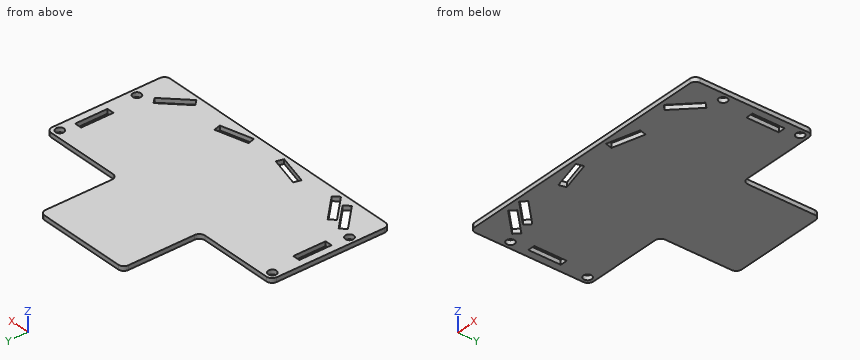
Autodesk Inventor part; units mm, degrees
ref_plane "YZ Plane" through (0, 0, 0) normal (1, 0, 0) x (0, 1, 0)
ref_plane "XZ Plane" through (0, 0, 0) normal (0, 1, 0) x (-1, 0, 0)
ref_plane "XY Plane" through (0, 0, 0) normal (0, 0, 1) x (1, 0, 0)
sketch "Szkic1" plane through (0, 0, 0) normal (0, 0, 1) x (1, 0, 0)
  circle A0 centre (-2, -7.4599) radius 1.4
  circle A1 centre (-2, 20.4244) radius 1.4
  circle A2 centre (-95, -7.4599) radius 1.4
  circle A3 centre (-95, 20.4244) radius 1.4
  line L0 (-98.5, 23.9244) -> (-98.5, -20.9244)
  line L1 (-97.6, 23.9244) -> (-97.6, -20.9244)
  line L2 (-98.5, -20.9244) -> (-91.5, -20.9244)
  line L3 (-98.5, 23.9244) -> (-91.5, 23.9244)
  line L4 (-98.5, -19.9244) -> (-91.5, -19.9244)
  line L5 (-91.5, -7.4599) -> (-91.5, -20.9244)
  line L6 (-97.6, 23.0244) -> (-92.3999, 23.0244)
  line L7 (-48.5, -51.6271) -> (-48.5, 68.0164)
  line L8 (-97.6, -19.9244) -> (-48.5, -19.9244)
  line L9 (-48.5, -19.9244) -> (-48.5, 23.0244)
  line L10 (-48.5, 23.0244) -> (-97.6, 23.0244)
  line L11 (-97.6, 23.0244) -> (-97.6, -19.9244)
  line L12 (0.6, -19.9244) -> (-48.5, -19.9244)
  line L13 (-48.5, 23.0244) -> (0.6, 23.0244)
  line L14 (0.6, 23.0244) -> (0.6, -19.9244)
  point P0 (0, 0)
  dimension "d0" = 0.9
  dimension "d1" = 1
  dimension "d2" = 0.9
extrude "Wyciągnięcie proste1" add sketch "Szkic1" along normal blind 1.6 contours L1 L6 L10 L7 L8 L4 | L7 L13 L14 L12
sketch "Szkic2" plane through (0, 0, 1.6) normal (0, 0, 1) x (1, 0, 0)
  line L0 (-29.5, 25.9244) -> (-29.5, 36.1286)
  line L1 (-31.5, 51.9244) -> (-65.5, 51.9244)
  line L2 (-67.5, 36.1286) -> (-67.5, 25.9244)
  line L3 (0.6, 23.0244) -> (-97.6, 23.0244)
  line L4 (-29.5, 23.0244) -> (-67.5, 23.0244)
  line L5 (-67.5, 23.0244) -> (-67.5, 51.9244)
  line L6 (-67.5, 51.9244) -> (-29.5, 51.9244)
  line L7 (-29.5, 51.9244) -> (-29.5, 23.0244)
  line L8 (-30.4, 23.9244) -> (-66.6, 23.9244)
  line L9 (-66.6, 23.9244) -> (-66.6, 51.0244)
  line L10 (-66.6, 51.0244) -> (-30.4, 51.0244)
  line L11 (-30.4, 51.0244) -> (-30.4, 23.9244)
  line L12 (-30.4, 23.9244) -> (-30.4, 23.0244)
  line L13 (-66.6, 23.9244) -> (-66.6, 23.0244)
  point P0 (0, 0)
  point P1 (-67.5, 37.4744)
  point P2 (-29.5, 37.4744)
  point P3 (-29.5, 31.0265)
  point P4 (-48.5, 51.9244)
  dimension "d5" = 0.9
extrude "Wyciągnięcie proste2" add sketch "Szkic2" against normal blind 1.6 contours L3 L13 L8 L12 | L8 L9 L10 L11
sketch "Szkic3" plane through (0, 0, 1.6) normal (0, 0, 1) x (1, 0, 0)
  line L0 (-94.4, -0.5756) -> (-94.4, 10.1244)
  line L1 (-94.4, 10.1244) -> (-92.8, 10.1244)
  line L2 (-92.8, 10.1244) -> (-92.8, -0.5756)
  line L3 (-94.4, -0.5756) -> (-92.8, -0.5756)
  line L4 (-77.7433, -17.9244) -> (-76.6119, -16.7931)
  line L5 (-77.7433, -17.9244) -> (-85.3094, -10.3584)
  line L6 (-84.178, -9.227) -> (-76.6119, -16.7931)
  line L7 (-85.3094, -10.3584) -> (-84.178, -9.227)
  line L8 (-63.3019, -13.6096) -> (-52.9665, -16.379)
  line L9 (-63.716, -15.1551) -> (-63.3019, -13.6096)
  line L10 (-53.3806, -17.9244) -> (-63.716, -15.1551)
  line L11 (-29.1305, -15.1551) -> (-39.4659, -17.9244)
  line L12 (-39.88, -16.379) -> (-29.5446, -13.6096)
  line L13 (-29.1305, -15.1551) -> (-29.5446, -13.6096)
  line L14 (-39.4659, -17.9244) -> (-39.88, -16.379)
  line L15 (-53.3806, -17.9244) -> (-52.9665, -16.379)
  line L16 (-14.4607, -17.9244) -> (-15.592, -16.7931)
  line L17 (-15.592, -16.7931) -> (-8.026, -9.227)
  line L18 (-6.8946, -10.3584) -> (-14.4607, -17.9244)
  line L19 (-6.8946, -10.3584) -> (-8.026, -9.227)
  line L20 (-2.6, 14.4244) -> (-4.2, 14.4244)
  line L21 (-4.2, 3.7244) -> (-4.2, 14.4244)
  line L22 (-2.6, 3.7244) -> (-4.2, 3.7244)
  line L23 (-2.6, 14.4244) -> (-2.6, 3.7244)
  line L24 (-92.3, -1.0756) -> (-92.3, 10.6244)
  line L25 (-92.3, 10.6244) -> (-94.9, 10.6244)
  line L26 (-94.9, 10.6244) -> (-94.9, -1.0756)
  line L27 (-94.9, -1.0756) -> (-92.3, -1.0756)
  line L28 (-75.9048, -16.7931) -> (-77.7433, -18.6316)
  line L29 (-77.7433, -18.6316) -> (-86.0165, -10.3584)
  line L30 (-86.0165, -10.3584) -> (-84.178, -8.5199)
  line L31 (-84.178, -8.5199) -> (-75.9048, -16.7931)
  line L32 (-52.3541, -16.0254) -> (-63.6554, -12.9972)
  line L33 (-63.6554, -12.9972) -> (-64.3284, -15.5086)
  line L34 (-64.3284, -15.5086) -> (-53.027, -18.5368)
  line L35 (-53.027, -18.5368) -> (-52.3541, -16.0254)
  line L36 (-29.1911, -12.9972) -> (-40.4924, -16.0254)
  line L37 (-40.4924, -16.0254) -> (-39.8195, -18.5368)
  line L38 (-39.8195, -18.5368) -> (-28.5181, -15.5086)
  line L39 (-28.5181, -15.5086) -> (-29.1911, -12.9972)
  line L40 (-8.026, -8.5199) -> (-16.2991, -16.7931)
  line L41 (-16.2991, -16.7931) -> (-14.4607, -18.6316)
  line L42 (-14.4607, -18.6316) -> (-6.1875, -10.3584)
  line L43 (-6.1875, -10.3584) -> (-8.026, -8.5199)
  line L44 (-4.7, 3.2244) -> (-4.7, 14.9244)
  line L45 (-4.7, 14.9244) -> (-2.1, 14.9244)
  line L46 (-2.1, 14.9244) -> (-2.1, 3.2244)
  line L47 (-2.1, 3.2244) -> (-4.7, 3.2244)
  point P0 (0, 0)
  dimension "d8" = 0.5
  dimension "d9" = 0.5
  dimension "d10" = 0.5
  dimension "d11" = 0.5
  dimension "d12" = 0.5
  dimension "d13" = 0.5
extrude "Wyciągnięcie proste3" cut sketch "Szkic3" against normal blind 1.6 contours L0 L1 L2 L3 | L5 L7 L6 L4 | L8 L15 L10 L9 | L11 L14 L12 L13 | L16 L17 L19 L18 | L23 L22 L21 L20 | L27 L26 L25 L24 | L28 L29 L30 L31 | L35 L34 L33 L32 | L39 L38 L37 L36 | L43 L42 L41 L40 | L44 L45 L46 L47
fillet "Zaokrąglenie1" radius 2 8 edges at (-66.6, 51.0244, 0.8) (-66.6, 23.0244, 0.8) (-97.6, 23.0244, 0.8) (-97.6, -19.9244, 0.8) (0.6, 23.0244, 0.8) (0.6, -19.9244, 0.8) (-30.4, 23.0244, 0.8) (-30.4, 51.0244, 0.8)
sketch "Szkic4" plane through (0, 0, 1.6) normal (0, 0, 1) x (1, 0, 0)
  circle A0 centre (-2, 20.4244) radius 1.4
  circle A1 centre (-2, -7.4599) radius 1.4
  circle A2 centre (-95, 20.4244) radius 1.4
  circle A3 centre (-95, -7.4599) radius 1.4
  point P0 (0, 0)
hole "Otwór1" at (-2, 20.4244, 1.6) at (-2, -7.4599, 1.6) at (-95, 20.4244, 1.6) at (-95, -7.4599, 1.6) direction (0, 0, -1) diameter 3 end through all
sketch "Szkic5" plane through (0, 0, 1.6) normal (0, 0, 1) x (1, 0, 0)
  circle A0 centre (-95, 20.4244) radius 1.5
  circle A1 centre (-2, 20.4244) radius 1.5
  circle A2 centre (-2, -7.4599) radius 1.5
  circle A3 centre (-95, -7.4599) radius 1.5
  arc A4 (-30.4, 49.0244) -> (-32.4, 51.0244) centre (-32.4, 49.0244) ccw
  line L0 (-32.4, 51.0244) -> (-64.6, 51.0244)
  arc A5 (-64.6, 51.0244) -> (-66.6, 49.0244) centre (-64.6, 49.0244) ccw
  line L1 (-66.6, 49.0244) -> (-66.6, 25.0244)
  arc A6 (-68.6, 23.0244) -> (-66.6, 25.0244) centre (-68.6, 25.0244) ccw
  line L2 (-68.6, 23.0244) -> (-95.6, 23.0244)
  arc A7 (-95.6, 23.0244) -> (-97.6, 21.0244) centre (-95.6, 21.0244) ccw
  line L3 (-97.6, 21.0244) -> (-97.6, -17.9244)
  arc A8 (-97.6, -17.9244) -> (-95.6, -19.9244) centre (-95.6, -17.9244) ccw
  line L4 (-95.6, -19.9244) -> (-1.4, -19.9244)
  arc A9 (-1.4, -19.9244) -> (0.6, -17.9244) centre (-1.4, -17.9244) ccw
  line L5 (0.6, -17.9244) -> (0.6, 21.0244)
  arc A10 (0.6, 21.0244) -> (-1.4, 23.0244) centre (-1.4, 21.0244) ccw
  line L6 (-1.4, 23.0244) -> (-28.4, 23.0244)
  arc A11 (-30.4, 25.0244) -> (-28.4, 23.0244) centre (-28.4, 25.0244) ccw
  line L7 (-30.4, 25.0244) -> (-30.4, 49.0244)
  line L8 (-94.9, -1.0756) -> (-94.9, 10.6244)
  line L9 (-94.9, 10.6244) -> (-92.3, 10.6244)
  line L10 (-92.3, 10.6244) -> (-92.3, -1.0756)
  line L11 (-92.3, -1.0756) -> (-94.9, -1.0756)
  line L12 (-6.1875, -10.3584) -> (-14.4607, -18.6316)
  line L13 (-14.4607, -18.6316) -> (-16.2991, -16.7931)
  line L14 (-16.2991, -16.7931) -> (-8.026, -8.5199)
  line L15 (-8.026, -8.5199) -> (-6.1875, -10.3584)
  line L16 (-28.5181, -15.5086) -> (-39.8195, -18.5368)
  line L17 (-39.8195, -18.5368) -> (-40.4924, -16.0254)
  line L18 (-40.4924, -16.0254) -> (-29.1911, -12.9972)
  line L19 (-29.1911, -12.9972) -> (-28.5181, -15.5086)
  line L20 (-77.7433, -18.6316) -> (-86.0165, -10.3584)
  line L21 (-86.0165, -10.3584) -> (-84.178, -8.5199)
  line L22 (-84.178, -8.5199) -> (-75.9048, -16.7931)
  line L23 (-75.9048, -16.7931) -> (-77.7433, -18.6316)
  line L24 (-4.7, 14.9244) -> (-2.1, 14.9244)
  line L25 (-2.1, 14.9244) -> (-2.1, 3.2244)
  line L26 (-2.1, 3.2244) -> (-4.7, 3.2244)
  line L27 (-4.7, 3.2244) -> (-4.7, 14.9244)
  line L28 (-53.027, -18.5368) -> (-64.3284, -15.5086)
  line L29 (-64.3284, -15.5086) -> (-63.6554, -12.9972)
  line L30 (-63.6554, -12.9972) -> (-52.3541, -16.0254)
  line L31 (-52.3541, -16.0254) -> (-53.027, -18.5368)
  line L32 (-91.5, -9.7839) -> (-83.2269, -18.057)
  line L33 (-83.2269, -18.057) -> (-81.3884, -16.2185)
  line L34 (-81.3884, -16.2185) -> (-89.6615, -7.9454)
  line L35 (-89.6615, -7.9454) -> (-91.5, -9.7839)
  line L36 (-91.5, -7.4599) -> (-91.5, -20.9244)
  line L37 (-77.7433, -18.057) -> (-77.7433, -19.9244) construction
  line L38 (-83.2269, -18.057) -> (-83.2269, -19.9244) construction
  point P0 (0, 0)
extrude "Wyciągnięcie proste4" cut sketch "Szkic5" against normal through all contours L35 L34 L33 L32
properties part number "main_pcb"
Part model, mm, in its own coordinate system. Round coordinates to 2 decimals unless told otherwise and drop trailing zeros. Loops run counter-clockwise (first coordinate to the right, second up) from the corner with the lowest first, then second, coordinate; pieces in that order, holes last. Notation, with made-up numbers: (-15.75, 71) - (-6.75, 71) arc R15 ccw to (-6.75, 96) - close; hole circle Ø2 at (41.5, 26.5). An arc over 180 degrees is marked (long way). Answer as a JSON object with one key per item and string values.
Item 1: Band-saw the part on A-A on x = -10. List the corners of the cut face in (y, z), plus the area to 3 significant figures.
Output:
{"outline": "(-19.92, 0) - (-14.17, 0) - (-14.17, 1.6) - (-19.92, 1.6) - close; (-10.49, 0) - (23.02, 0) - (23.02, 1.6) - (-10.49, 1.6) - close", "area": "62.8 mm2"}
Item 2: Band-saw the part on C-C on z = 1.15. State how many separate pieces and enclosed holes the cut face has, plus the area to 3 significant figures.
Output:
{"separate pieces": "1", "enclosed holes": "11", "area": "4,990 mm2"}
Item 3: Band-saw the part on B-B on y = -11.5. List the corners of the cut face in (x, z).
Output:
{"outline": "(-97.6, 0) - (-89.78, 0) - (-89.78, 1.6) - (-97.6, 1.6) - close; (-86.11, 0) - (-84.87, 0) - (-84.87, 1.6) - (-86.11, 1.6) - close; (-81.2, 0) - (-11.01, 0) - (-11.01, 1.6) - (-81.2, 1.6) - close; (-7.33, 0) - (0.6, 0) - (0.6, 1.6) - (-7.33, 1.6) - close"}
Item 4: Wall check: L1, parallel to X at y = 4, z = 1.55; L2, parallel to Y at x = -95, z = 1.25; L3, parallel to X at y = 0, z = 1.2. Give the ranges that are in metal, low to high.
Output:
{"L1": "-97.6 to -94.9, -92.3 to -4.7, -2.1 to 0.6", "L2": "-19.92 to -8.96, -5.96 to 18.92, 21.92 to 23.02", "L3": "-97.6 to -94.9, -92.3 to 0.6"}
Item 5: Band-saw the part on D-D on y = 40.5. List the corners of the cut face in (x, z), plus the area to 3 significant figures.
Output:
{"outline": "(-66.6, 0) - (-30.4, 0) - (-30.4, 1.6) - (-66.6, 1.6) - close", "area": "57.9 mm2"}
Item 6: Pin check, flat tips, straight feed: pin 1 (0.8 mm diameter, centred on x = -94, z = 1, fed in from +Y); pin 2 (0.8 mm diameter, centred on y = 34.5, z = 1, fed in from +X); pin 3 (1.8 mm diameter, centred on x = -2, y = -7.46, fed in from +Z). Stop position of each tip, or through.
Output:
{"pin 1": "y = 23.02", "pin 2": "x = -30.4", "pin 3": "through"}
